Read the model definition and answer for the solid it produces. Units are mm, in the model's axes. A direction names the side the tool comes from. Coordinates: 2 decimals unless noted, no trailing zeros. Return JSON: item names as keys, results as strings.
```python
from build123d import *

# Parameters (mm, degrees)
F0_R     = 6
F3_R     = 2.5
F4_DEPTH = 2
F5_DEPTH = 2


with BuildPart() as f2:
    # F2: sweep along a path in F1
    with BuildLine(Plane.XZ) as f2_path:
        ThreePointArc((6, 0), (-2.493903, 20.506097), (-23, 29))
        Line((-23, 29), (-32.231277, 29))
        Line((-32.231277, 29), (-41.462554, 29))
        ThreePointArc((-41.462554, 29), (-61.96865, 20.506097), (-70.462554, 0))
    # F0 (on Top) → F2 (sweep)
    with BuildSketch(Plane.XY):
        Circle(F0_R)
    sweep(path=f2_path.line)

    # F3 (on face) → F4 (cut)
    with BuildSketch(Plane(origin=(0, 0, 0), x_dir=(1, 0, 0), z_dir=(0, 0, -1))):
        with Locations((-64.462554, 0)):
            Circle(F3_R)
    extrude(amount=-F4_DEPTH, mode=Mode.SUBTRACT)

    # F3 (on face) → F5 (cut)
    with BuildSketch(Plane(origin=(0, 0, 0), x_dir=(1, 0, 0), z_dir=(0, 0, -1))):
        Circle(F3_R)
    extrude(amount=-F5_DEPTH, mode=Mode.SUBTRACT)


solid = f2.part
```
(1) Determine the mould class of faces 1 (the face through (-66.446, 1.521, 0.986)), 2 (the face through (-0.54, 2.44, 0.99)), 3 (the face through (-64, -3, 0)) for opening direction X: +X half, -X half, draft (parallel to the pull), parting line (faces both ways), or undercut.
Answer:
{"face 1": "undercut", "face 2": "undercut", "face 3": "draft"}
(2) Which of the six approach directions +Z, -Z, +X, -X, +Y, -Y give full straight-line access (tool end or side, diameter ignored) to faces 4 (the face through (3, 0, 0)), 5 (the face through (0, 0, 2))?
Answer:
{"face 4": "-Z, +X, -X, +Y, -Y", "face 5": "-Z"}
(3) Straight lines are drawn through the part: line 1 (X direction, y = -2, z = 8); line 2 (X direction, y = -5, z = 9.25); line 3 (Z direction, x = -3, y = -0.25). For each, find the intervals that lie inside material, in ascending order. Write a range as from..to.
Answer:
{"line 1": "-68.98..-56.85, -7.61..4.52", "line 2": "-66.1..-58.84, -5.63..1.64", "line 3": "0..20.99"}
(4) Flat-ended cylindrical pins translate along their axes: P1, Ø2, axis at x = -48.5, y = -4, coming from the -Z side; P2, Ø5, axis at x = -28.5, z = 26, coming from the +Y side; P3, Ø1.5, axis at y = -2, z = 8.5, coming from the -X side; P4, Ø5, axis at x = -23.5, z = 24.5, coming from the -Y side. Find the tip coordinate at first contact, or state that the pin passes through.
Answer:
{"P1": "z = 16.22", "P2": "y = 5.98", "P3": "x = -69.16", "P4": "y = -6"}
